from build123d import *

# Parameters (mm, degrees)
SKETCH_W       = 31.75
SKETCH_H       = 31.75
SKETCH_W_2     = 26.2128
SKETCH_H_2     = 26.2128
PAD_DEPTH      = 609.6
PAD_DEPTH_BACK = 609.6
POCKET_DEPTH   = 31.75


with BuildPart() as part:
    # Sketch → Pad (new body, two sides)
    with BuildSketch(Plane.YZ) as pad_sk:
        Rectangle(SKETCH_W, SKETCH_H)
        Rectangle(SKETCH_W_2, SKETCH_H_2, mode=Mode.SUBTRACT)
    extrude(amount=PAD_DEPTH)
    extrude(pad_sk.sketch, amount=-PAD_DEPTH_BACK)

    # Sketch001 → Pocket (cut)
    with BuildSketch(Plane(origin=(0, 0, 15.875), x_dir=(0, -1, 0), z_dir=(0, 0, 1))):
        Polygon((15.875, 609.6), (-15.875, 609.6), (15.875, 577.85), align=None)
    pocket = extrude(amount=-POCKET_DEPTH, mode=Mode.SUBTRACT)

    # Mirrored: Pocket across Sketch001 H_Axis
    add(pocket.mirror(Plane(origin=(0, 0, 15.875), x_dir=(0, 0, 1), z_dir=(1, 0, 0))), mode=Mode.SUBTRACT)


solid = part.part
Build history of the part. All positions in model axes, mm. A direction names the side the tool comes from. Round coordinates to 2 decimals unless told otherwise and drop trailing zeros. Loops run counter-clockwise (first coordinate to the right, second up) from the corner with the lowest first, then second, coordinate; pieces in that order, holes last. Notation, with made-up numbers: (82.25, 3) -> (123.25, 3) arc R25 ccw to (123.25, 40) -> close; hole circle Ø3 at (50, 22). An arc over 180 degrees is marked (long way). Answer in a Markdown table with one row per item.
Item 1: Saw through at B-B (z = -5). Write the cut outline in (x, y) (3 decimals).
Answers below:
| item | result |
|---|---|
| outline | (-609.6, 15.875) -> (-606.831, 13.106) -> (606.831, 13.106) -> (609.6, 15.875) -> close; (-580.619, -13.106) -> (-577.85, -15.875) -> (577.85, -15.875) -> (580.619, -13.106) -> close |
Item 2: Which spindle directions (+Z, -Z, +X, -X, +Y, -Y) get a long thin tool onto all of the face, cutting with end or side? Do faces 5 (the flat face through (8, 0, -13.106)), 6 (the flat face through (8, -15.875, 0)). Say none if no direction does.
Answers below:
| item | result |
|---|---|
| face 5 | +X, -X |
| face 6 | +Z, -Z, +X, -X, -Y |
Item 3: Saw through at C-C (y = 8). Write the cut outline in (x, z) (3 decimals), and give its area (3 significant figures).
Answers below:
| item | result |
|---|---|
| outline | (-601.725, -15.875) -> (601.725, -15.875) -> (601.725, -13.106) -> (-601.725, -13.106) -> close; (-601.725, 13.106) -> (601.725, 13.106) -> (601.725, 15.875) -> (-601.725, 15.875) -> close |
| area | 6,660 mm² |
Item 4: Saw through at A-A (x = -147.5). Write the cut outline in (y, z) (3 decimals).
Answers below:
| item | result |
|---|---|
| outline | (-15.875, -15.875) -> (15.875, -15.875) -> (15.875, 15.875) -> (-15.875, 15.875) -> close; hole (-13.106, -13.106) -> (13.106, -13.106) -> (13.106, 13.106) -> (-13.106, 13.106) -> close |
Item 5: Mould opens along Z. For faces 1 (the flat face through (8, -13.106, 0)), 2 (the flat face through (8, 0, 13.106)), 3 (the flat face through (9, 0, 15.875)), 4 (the flat face through (-593.947, 0.222, -13.889)) say: +Z half, -Z half, draft (parallel to the pull), parting line (faces both ways), or undercut.
Answers below:
| item | result |
|---|---|
| face 1 | undercut |
| face 2 | undercut |
| face 3 | +Z half |
| face 4 | draft |
Item 6: Pin check, flat tips, straight feed: pin 1 (8 mm diameter, centred on y = 10.5, z = -4.5, fed in from -X) (3 decimals); pin 2 (10 mm diameter, centred on y = -8.5, z = -10.5, fed in from -X). Stop position of each tip, or through.
Answers below:
| item | result |
|---|---|
| pin 1 | stops at x = -608.225 |
| pin 2 | stops at x = -589.49 |
Item 7: Drill centre lines: L1, parallel to Z at x = 131, y = 6 (3 decimals); L2, parallel to X at y = 13.5, z = -11.5 (3 decimals). Where is each one in solid material? Low to high. Write a range as [from, to].
Answers below:
| item | result |
|---|---|
| L1 | z = [-15.875, -13.106], [13.106, 15.875] |
| L2 | x = [-607.225, 607.225] |
